from build123d import *

# Parameters (mm, degrees)
F1_DEPTH  = 35
F3_DEPTH  = 15
F4_D      = 3.2
F5_DEPTH  = 1
F6_R      = 3
F7_DEPTH  = 55.001
F13_DEPTH = 11


with BuildPart() as f1:
    # F0 (on Top) → F1 (new body)
    with BuildSketch(Plane.XY):
        with BuildLine():
            Line((27.5, 5.35), (27.5, 7.5))
            Line((27.5, 7.5), (-27.5, 7.5))
            Line((-27.5, 7.5), (-27.5, -7.5))
            Line((-27.5, -7.5), (27.5, -7.5))
            Line((27.5, -7.5), (27.5, -5.35))
            Line((27.5, -5.35), (17.1071307506, -5.35))
            ThreePointArc((17.1071307506, -5.35), (9.25, 0), (17.1071307506, 5.35))
            Line((17.1071307506, 5.35), (27.5, 5.35))
        make_face()
    extrude(amount=F1_DEPTH)

    # F2 (on face) → F3 (cut, through all)
    with BuildSketch(Plane.XZ.offset(7.5)):
        with BuildLine():
            Line((-17.5, 35), (-17.5, 23.6602540378))
            ThreePointArc((-17.5, 23.6602540378), (-12.5, 5), (-7.5, 23.6602540378))
            Line((-7.5, 23.6602540378), (-7.5, 35))
            Line((-7.5, 35), (-17.5, 35))
        make_face()
    extrude(amount=-F3_DEPTH, mode=Mode.SUBTRACT)

    # F4 (through all)
    with Locations(Plane.XZ.offset(7.5)):
        with Locations((23, 28), (23, 7)):
            Hole(F4_D / 2)

    # F2 (on face) → F5 (cut)
    with BuildSketch(Plane.XZ.offset(7.5)):
        Polygon((25.75, 29.5877132403), (23, 31.1754264805), (20.25, 29.5877132403), (20.25, 26.4122867597), (23, 24.8245735195), (25.75, 26.4122867597), align=None)
        Polygon((25.75, 8.5877132403), (23, 10.1754264805), (20.25, 8.5877132403), (20.25, 5.4122867597), (23, 3.8245735195), (25.75, 5.4122867597), align=None)
    extrude(amount=-F5_DEPTH, mode=Mode.SUBTRACT)

    # F6 (on face) → F7 (cut, through all)
    with BuildSketch(Plane(origin=(-27.5, 0, 0), x_dir=(0, -1, 0), z_dir=(-1, 0, 0))):
        with Locations((0, 30)):
            Circle(F6_R)
    extrude(amount=-F7_DEPTH, mode=Mode.SUBTRACT)

    # F12 (on offset) → F13 (cut)
    with BuildSketch(Plane(origin=(12.25, 0, 0), x_dir=(0, -1, 0), z_dir=(-1, 0, 0))):
        Polygon((0, 35.6869001515), (-4.925, 32.8434500758), (-4.925, 27.1565499242), (0, 24.3130998485), (4.925, 27.1565499242), (4.925, 32.8434500758), align=None)
    extrude(amount=F13_DEPTH, mode=Mode.SUBTRACT)


solid = f1.part
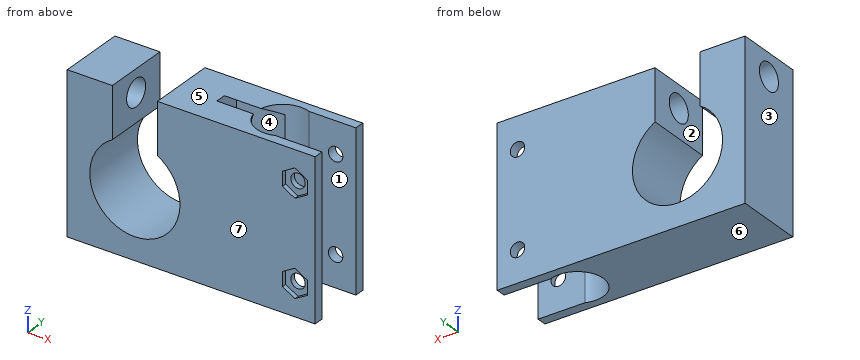
Source: CAD feature listing. Evaluate the final solid. Frame: model axes, mm. Face numbers are marked on the shaded views. A direction names the side the tool comes from. Coordinates: 2 decimals unless noted, no trailing zeros. Write each loop counter-clockwise with the first axis right and the second up, starting at its lowest first coordinate (ties: lowest second). Pieces come first, ordered by that corner, then holes. Notation, with made-up numbers: M -29.5,23.5 L -8.5,23.5 A36 ccw -8.5,62.5 Z; hole C -26.75,-27 d7. An arc over 180 degrees is marked long. Use a Markdown table: item, result.
1) First-contact query: pin 1 Ø9 at (y, z) = (-0.5, 29.5) entering from +X; pin 2 Ø4 at (x, y) = (-11, -4) entering from -Z; pin 3 Ø2 at (y, z) = (2.5, 28) entering from +X. Flat tips, straight axial feed; report the tip coordinate or a pass-through.
Conclusion:
| item | result |
|---|---|
| pin 1 | stops at x = 12.16 |
| pin 2 | stops at z = 0 |
| pin 3 | stops at x = 1.25 |
2) Reachability of the marked faces 1, 2 and 3 from +Z, -Z, +X, -X, +Y, -Y: full face, straight path, thin tool, end or side. Return the list, or none.
Conclusion:
| item | result |
|---|---|
| face 1 | +Z, -Z, +X |
| face 2 | +Z, +Y, -Y |
| face 3 | +Z, -Z, -X, +Y, -Y |
3) Section A-A, the plane z = 7. Output: boundary loops of the cut face in (x, y).
Conclusion:
| item | result |
|---|---|
| outline | M -27.5,-7.5 L -18.5,-7.5 L -18.5,7.5 L -27.5,7.5 Z; M -6.5,-7.5 L 20.25,-7.5 L 20.25,-6.5 L 21.4,-6.5 L 21.4,-5.35 L 17.11,-5.35 A5.75 cw long 17.11,5.35 L 21.4,5.35 L 21.4,7.5 L -6.5,7.5 Z; M 24.6,-6.5 L 25.75,-6.5 L 25.75,-7.5 L 27.5,-7.5 L 27.5,-5.35 L 24.6,-5.35 Z; M 24.6,5.35 L 27.5,5.35 L 27.5,7.5 L 24.6,7.5 Z |
4) Ray query, L1, parallel to Z at x = 23, y = -5.6; L2, parallel to Y at x = 20, z = 3.5; L3, parallel to Y at x = 15, z = 14. Return the intervals inside material, ascending.
Conclusion:
| item | result |
|---|---|
| L1 | z = 0 to 5.4, 8.6 to 26.4, 29.6 to 35 |
| L2 | y = -7.5 to -5.35, 5.35 to 7.5 |
| L3 | y = -7.5 to -5.75, 5.75 to 7.5 |
5) Section B-B, the plane x = 19. Output: boundary loops of the cut face in (y, z).
Conclusion:
| item | result |
|---|---|
| outline | M -7.5,0 L -5.35,0 L -5.35,35 L -7.5,35 Z; M 5.35,0 L 7.5,0 L 7.5,35 L 5.35,35 Z |
6) Section D-D, the plane z = 25.5. Output: boundary loops of the cut face in (x, y), then the cut area to 3 significant figures.
Conclusion:
| item | result |
|---|---|
| outline | M -27.5,-7.5 L -17.5,-7.5 L -17.5,7.5 L -27.5,7.5 Z; M -7.5,-7.5 L 21.83,-7.5 L 21.83,-6.5 L 24.17,-6.5 L 24.17,-7.5 L 27.5,-7.5 L 27.5,-5.35 L 17.11,-5.35 A5.75 cw 9.63,-2.06 L 1.25,-2.06 L 1.25,2.06 L 9.63,2.06 A5.75 cw 17.11,5.35 L 27.5,5.35 L 27.5,7.5 L -7.5,7.5 Z |
| area | 452 mm^2 |
7) Mould query, pull axis Z, two halves, no side actions, for the marked faces 4, 5, 6 and 7. Classes: pulls with the +Z half, pulls with the -Z half, needs draft (parallel to the pull), parting line crosses it, or undercut.
Conclusion:
| item | result |
|---|---|
| face 4 | undercut |
| face 5 | pulls with the +Z half |
| face 6 | pulls with the -Z half |
| face 7 | needs draft |
8) Section C-C, the plane y = 2. Output: boundary loops of the cut face in (x, z).
Conclusion:
| item | result |
|---|---|
| outline | M -27.5,0 L 9.61,0 L 9.61,25.47 L 1.25,25.47 L 1.25,27.76 L -7.5,27.76 L -7.5,23.66 A10 cw long -17.5,23.66 L -17.5,27.76 L -27.5,27.76 Z; M -27.5,32.24 L -17.5,32.24 L -17.5,35 L -27.5,35 Z; M -7.5,32.24 L 1.25,32.24 L 1.25,34.53 L 9.61,34.53 L 9.61,35 L -7.5,35 Z |
